```python
from build123d import *

# Parameters (mm, degrees)
PAD_DEPTH           = 0.8
PAD001_DEPTH        = 6.1
PAD002_DEPTH        = 5.7
POCKET_DEPTH        = 5.7
PAD003_PROFILE_R    = 1.45
PAD003_DEPTH        = 5.7
POCKET001_PROFILE_R = 1.05
POCKET001_DEPTH     = 12.6
POCKET002_PROFILE_W = 2.5
POCKET002_PROFILE_H = 2.5
POCKET002_DEPTH     = 6.1


with BuildPart() as part:
    # Sketch → Pad (new body)
    with BuildSketch(Plane.XY):
        Polygon((-6.1, 4.4), (6.1, 4.4), (6.1, -4.4), (-3.1, -4.4), (-6.1, -1.9), align=None)
    extrude(amount=PAD_DEPTH)

    # Pad001_Profile → Pad001 (join)
    with BuildSketch(Plane(origin=(0.115466, 0.066286, 0.8), x_dir=(0, 1, 0), z_dir=(0, 0, 1))):
        Polygon((3.633714, -5.984534), (3.633714, 6.215466), (-1.966286, 6.215466), (-3.766286, 4.115466), (-3.766286, -5.984534), align=None)
    extrude(amount=PAD001_DEPTH)

    # Pad002_Profile → Pad002 (join)
    with BuildSketch(Plane(origin=(0.266979, 0, 6.9), x_dir=(0, 1, 0), z_dir=(0, 0, 1))):
        with BuildLine():
            Line((3.45, -5.283021), (3.45, 2.516979))
            ThreePointArc((3.45, 2.516979), (0, 5.966979), (-3.45, 2.516979))
            Line((-3.45, 2.516979), (-3.45, -5.283021))
            Line((-3.45, -5.283021), (3.45, -5.283021))
        make_face()
    extrude(amount=PAD002_DEPTH)

    # Pocket_Profile → Pocket (cut)
    with BuildSketch(Plane(origin=(0.027606, 0, 12.6), x_dir=(0, 1, 0), z_dir=(0, 0, 1))):
        with BuildLine():
            Line((3.05, -4.722394), (3.05, 2.277606))
            ThreePointArc((3.05, 2.277606), (0, 5.327606), (-3.05, 2.277606))
            Line((-3.05, 2.277606), (-3.05, -4.722394))
            Line((-3.05, -4.722394), (3.05, -4.722394))
        make_face()
    extrude(amount=-POCKET_DEPTH, mode=Mode.SUBTRACT)

    # Pad003_Profile → Pad003 (join)
    with BuildSketch(Plane(origin=(2.3, 0, 6.9), x_dir=(0, 1, 0), z_dir=(0, 0, 1))):
        Circle(PAD003_PROFILE_R)
        with Locations((0, 4.1)):
            Circle(PAD003_PROFILE_R)
    extrude(amount=PAD003_DEPTH)

    # Pocket001_Profile → Pocket001 (cut)
    with BuildSketch(Plane(origin=(-1.8, 0, 12.6), x_dir=(0, 1, 0), z_dir=(0, 0, 1))):
        Circle(POCKET001_PROFILE_R)
        with Locations((0, -4.1)):
            Circle(POCKET001_PROFILE_R)
    extrude(amount=-POCKET001_DEPTH, mode=Mode.SUBTRACT)

    # Pocket002_Profile → Pocket002 (cut)
    with BuildSketch(Plane(origin=(2.3, 0, 6.1), x_dir=(0, 1, 0), z_dir=(0, 0, 1))):
        Rectangle(POCKET002_PROFILE_W, POCKET002_PROFILE_H)
        with Locations((0, 4.1)):
            Rectangle(POCKET002_PROFILE_W, POCKET002_PROFILE_H)
    extrude(amount=-POCKET002_DEPTH, mode=Mode.SUBTRACT)


solid = part.part
```
Design review of the part built by this model. Coordinates are the model's own, in mm. A direction names the side the tool comes from. Give positions to 0.01 mm unless a question says otherwise; leave off trailing zeros. Write each loop counter-clockwise with the first axis right and the second up, starting at its lowest first coordinate (ties: lowest second). Pieces come first, ordered by that corner, then holes. Notation, with made-up numbers: (85, 72) -> (143, 72) arc R29 cw to (143, 93) -> close; hole circle Ø5 at (21, 20). An arc over 180 degrees is marked (long way). Answer in a Markdown table with one row per item.
(1) Consider section D-D (x = 4). State the section outline as (y, z) points, then the cut area to 3 significant figures.
Results:
| item | result |
|---|---|
| outline | (-4.4, 0) -> (4.4, 0) -> (4.4, 0.8) -> (3.7, 0.8) -> (3.7, 6.9) -> (3.45, 6.9) -> (3.45, 12.6) -> (3.05, 12.6) -> (3.05, 6.9) -> (-3.05, 6.9) -> (-3.05, 12.6) -> (-3.45, 12.6) -> (-3.45, 6.9) -> (-3.7, 6.9) -> (-3.7, 0.8) -> (-4.4, 0.8) -> close |
| area | 56.7 mm2 |
(2) To check wall thickness, follow probe 1 along X at (y, z) = (0.5, 4); probe 2 along X at (y, z) = (0, 9); probe 3 along Y at (x, z) = (2.3, 8). State the ranges of each line that lie inside material, in increasing order.
Results:
| item | result |
|---|---|
| probe 1 | -6.1 to -3.05, -0.55 to 1.05, 3.55 to 6.1 |
| probe 2 | -5.7 to -5.3, -3.25 to -2.85, -0.75 to -0.35, 0.85 to 1.25, 3.35 to 3.75, 4.75 to 5.55 |
| probe 3 | -3.45 to -3.05, -1.45 to -1.05, 1.05 to 1.45, 3.05 to 3.45 |
(3) For faces 1 (the flat face through (4.75, 0, 10)), 2 (the flat face through (-3.05, 0, 3)), 3 (the flat face through (0, 3.7, 4)), list the 3-axis set-ups (+Z, -Z, +X, -X, +Y, -Y) from which the entire face can be reached by the end or side of a thin tool; tool diameter is ignored.
Results:
| item | result |
|---|---|
| face 1 | +Z |
| face 2 | -Z |
| face 3 | +Z, +X, -X, +Y |
(4) Mouldability with a two-part tool opening along X and no side actions: class faces 4 (the flat face through (-4.579, -3.167, 0.394)), 5 (the flat face through (5.55, 0, 10)), 6 (the flat face through (-2, 1.25, 3)) as +X half, -X half, draft (parallel to the pull), parting line (faces both ways), or undercut.
Results:
| item | result |
|---|---|
| face 4 | -X half |
| face 5 | +X half |
| face 6 | undercut |
(5) Consider section B-B (x = 2.3). State the section outline as (y, z) points.
Results:
| item | result |
|---|---|
| outline | (-4.4, 0) -> (-1.25, 0) -> (-1.25, 6.1) -> (-1.05, 6.1) -> (-1.05, 12.6) -> (-1.45, 12.6) -> (-1.45, 6.9) -> (-3.05, 6.9) -> (-3.05, 12.6) -> (-3.45, 12.6) -> (-3.45, 6.9) -> (-3.7, 6.9) -> (-3.7, 0.8) -> (-4.4, 0.8) -> close; (1.05, 6.1) -> (1.25, 6.1) -> (1.25, 0) -> (4.4, 0) -> (4.4, 0.8) -> (3.7, 0.8) -> (3.7, 6.9) -> (3.45, 6.9) -> (3.45, 12.6) -> (3.05, 12.6) -> (3.05, 6.9) -> (1.45, 6.9) -> (1.45, 12.6) -> (1.05, 12.6) -> close |
(6) Consider section A-A (z = 9.25). State the section outline as (x, y) points.
Results:
| item | result |
|---|---|
| outline | circle Ø2.9 at (-1.8, 0); (-2.25, -3.45) -> (5.55, -3.45) -> (5.55, 3.45) -> (-2.25, 3.45) arc R3.45 ccw to start; circle Ø2.9 at (2.3, 0); hole circle Ø2.1 at (-1.8, 0); hole (-2.25, -3.05) -> (4.75, -3.05) -> (4.75, 3.05) -> (-2.25, 3.05) arc R3.05 ccw to start; hole circle Ø2.1 at (2.3, 0) |
(7) Consider section C-C (z = 4.5). State the section outline as (x, y) points, then the cut area to 3 significant figures.
Results:
| item | result |
|---|---|
| outline | (-6.1, -1.9) -> (-4, -3.7) -> (6.1, -3.7) -> (6.1, 3.7) -> (-6.1, 3.7) -> close; hole (-3.05, -1.25) -> (-0.55, -1.25) -> (-0.55, 1.25) -> (-3.05, 1.25) -> close; hole (1.05, -1.25) -> (3.55, -1.25) -> (3.55, 1.25) -> (1.05, 1.25) -> close |
| area | 75.9 mm2 |
(8) Clearance check with flat-ended pins moving along their axes: pin 1 (6 mm diameter, centred on x = -3, z = 11.5, fed in from -Y); pin 2 (1.7 mm diameter, centred on x = 1, z = 8.5, fed in from +Y); pin 3 (1.2 mm diameter, centred on x = -1.5, y = 0.5, fed in from -Z). State where each tip first meets the part, or that it passes through.
Results:
| item | result |
|---|---|
| pin 1 | y = -3.45 |
| pin 2 | y = 3.45 |
| pin 3 | z = 6.1 |
